Part model, mm, in its own coordinate system. A direction names the side the tool comes from. Give positions to 0.01 mm unless a question says otherwise; leave off trailing zeros. Write each loop counter-clockwise with the first axis right and the second up, starting at its lowest first coordinate (ties: lowest second). Pieces come first, ordered by that corner, then holes.
from build123d import *

# Parameters (mm, degrees)
SKETCH1_W           = 93
SKETCH1_H           = 93
BOSS_EXTRUDE1_DEPTH = 80
SKETCH3_W           = 90
SKETCH3_H           = 90
CUT_EXTRUDE1_DEPTH  = 77
SKETCH4_W           = 35
SKETCH4_H           = 80
CUT_EXTRUDE2_DEPTH  = 5
FILLET1_R           = 10


with BuildPart() as part:
    # Sketch1 → Boss-Extrude1 (new body)
    with BuildSketch(Plane(origin=(0, 0, 0), x_dir=(1, 0, 0), z_dir=(0, 1, 0))):
        Rectangle(SKETCH1_W, SKETCH1_H)
    extrude(amount=BOSS_EXTRUDE1_DEPTH)

    # Sketch3 → Cut-Extrude1 (cut)
    with BuildSketch(Plane(origin=(0, 80, 0), x_dir=(1, 0, 0), z_dir=(0, 1, 0))):
        Rectangle(SKETCH3_W, SKETCH3_H)
    extrude(amount=-CUT_EXTRUDE1_DEPTH, mode=Mode.SUBTRACT)

    # Sketch4 → Cut-Extrude2 (cut)
    with BuildSketch(Plane.XY.offset(46.5)):
        with Locations((0, 40)):
            Rectangle(SKETCH4_W, SKETCH4_H)
    extrude(amount=-CUT_EXTRUDE2_DEPTH, mode=Mode.SUBTRACT)

    # Fillet1
    fillet1_edges = [part.edges().sort_by_distance(p)[0] for p in [
        (-17.5, 80, 45.75),
        (17.5, 80, 45.75),
    ]]
    fillet(fillet1_edges, radius=FILLET1_R)


solid = part.part
1) Saw through at A-A (x = 36). Write the cut outline in (y, z).
Check result:
outline: (0, -46.5) - (80, -46.5) - (80, -45) - (3, -45) - (3, 45) - (80, 45) - (80, 46.5) - (0, 46.5) - close
2) 3-axis set-ups, long thin cutter, end or side, ignore diameter. For faces 1 (the flat face through (-46.5, 39, 1)), 2 (the flat face through (31, 42, 45)), 3 (the flat face through (17.5, 32, 46)), 4 (the flat face through (46.5, 39, 1)), 5 (the cylindrical face through (20.51, 77.15, 45.74)): which of +Z, -Z, +X, -X, +Y, -Y reach the whole face in a straight line?
Check result:
face 1: +Z, -Z, -X, +Y, -Y
face 2: +Y
face 3: +Z, +Y, -Y
face 4: +Z, -Z, +X, +Y, -Y
face 5: +Z, +Y
3) Saw through at C-C (z = 26). Write the cut outline in (x, y).
Check result:
outline: (-46.5, 0) - (46.5, 0) - (46.5, 80) - (45, 80) - (45, 3) - (-45, 3) - (-45, 80) - (-46.5, 80) - close
4) Flat gauge pins, fed straight in: P1, Ø5, axis at x = 3, y = 8, coming from the +Z side; P2, Ø10, axis at x = -14.5, z = 35, coming from the +Y side; P3, Ø3.5, axis at x = -8.5, y = 2, coming from the +Z side. Where does each tip first touch, or does it go through?
Check result:
P1: stops at z = -45
P2: stops at y = 3
P3: stops at z = 41.5
5) Saw through at B-B (y = 37.5). Write the cut outline in (x, z), and give its area (4 significant figures).
Check result:
outline: (-46.5, -46.5) - (46.5, -46.5) - (46.5, 46.5) - (17.5, 46.5) - (17.5, 45) - (45, 45) - (45, -45) - (-45, -45) - (-45, 45) - (-17.5, 45) - (-17.5, 46.5) - (-46.5, 46.5) - close
area: 496.5 mm2
6) Drill centre lines: L1, parallel to X at y = 66, z = -25; L2, parallel to Y at x = -2, z = 3. Where is each one in solid material? Low to high.
Check result:
L1: x = -46.5 to -45, 45 to 46.5
L2: y = 0 to 3
7) Saw through at D-D (x = 14.5). Write the cut outline in (y, z).
Check result:
outline: (0, -46.5) - (80, -46.5) - (80, -45) - (3, -45) - (3, 41.5) - (0, 41.5) - close
8) Mould opens along Z. For faces 6 (the flat face through (-31, 42, 45)), 7 (the flat face through (-32, 39, 46.5)), 8 (the flat face through (45, 42, 1)), 9 (the flat face through (-1, 0, -1)) say: +Z half, -Z half, draft (parallel to the pull), parting line (faces both ways), or undercut.
Check result:
face 6: undercut
face 7: +Z half
face 8: undercut
face 9: draft
